Autodesk Inventor part; units mm, degrees
ref_plane "YZ Plane" through (0, 0, 0) normal (1, 0, 0) x (0, 1, 0)
ref_plane "XZ Plane" through (0, 0, 0) normal (0, 1, 0) x (-1, 0, 0)
ref_plane "XY Plane" through (0, 0, 0) normal (0, 0, 1) x (1, 0, 0)
sketch "Sketch2" plane through (0, 0, 0) normal (0, 1, 0) x (-1, 0, 0)
  line L0 (-30.2, -84) -> (30.2, -84)
  line L1 (30.2, -84) -> (30.2, 84)
  line L2 (30.2, 84) -> (-30.2, 84)
  line L3 (-30.2, 84) -> (-30.2, -84)
  line L4 (-30.2, -84) -> (30.2, 84) construction
  line L5 (30.2, -84) -> (-30.2, 84) construction
  point P0 (0, 0)
  dimension "d0" = 60.4
  dimension "d1" = 168
extrude "Extrusion1" add sketch "Sketch2" along normal blind 3
sketch "Sketch3" plane through (0, 3, 0) normal (0, 1, 0) x (1, 0, 0)
  line L0 (27.2, 81) -> (-27.2, 81)
  line L1 (-27.2, 81) -> (-27.2, -81)
  line L2 (-27.2, -81) -> (27.2, -81)
  line L3 (27.2, -81) -> (27.2, 81)
  line L4 (27.2, 81) -> (-27.2, -81) construction
  line L5 (-27.2, 81) -> (27.2, -81) construction
  line L6 (-30.2, 84) -> (-30.2, -84)
  line L7 (-30.2, -84) -> (30.2, -84)
  line L8 (24.2, 78) -> (-24.2, 78)
  line L9 (-24.2, 78) -> (-24.2, -78)
  line L10 (-24.2, -78) -> (24.2, -78)
  line L11 (24.2, -78) -> (24.2, 78)
  line L12 (24.2, 78) -> (-24.2, -78) construction
  line L13 (-24.2, 78) -> (24.2, -78) construction
  point P0 (0, 0)
  dimension "d4" = 3
  dimension "d5" = 3
  dimension "d6" = 3
  dimension "d7" = 3
extrude "Extrusion2" add sketch "Sketch3" along normal blind 30
fillet "Fillet1" radius 2 8 edges at (27.2, 18, 81) (-27.2, 18, 81) (-30.2, 1.5, 84) (30.2, 1.5, 84) (27.2, 18, -81) (-27.2, 18, -81) (30.2, 1.5, -84) (-30.2, 1.5, -84)
sketch "Sketch10" plane through (0, 3, 0) normal (0, 1, 0) x (1, 0, 0)
  line L0 (24.2, 78) -> (-24.2, 78)
  line L1 (-24.2, 78) -> (-24.2, -78)
  line L2 (-24.2, -78) -> (24.2, -78)
  line L3 (24.2, -78) -> (24.2, 78)
  line L4 (-24.2, -78) -> (24.2, -78)
  line L5 (24.2, -78) -> (24.2, -73.8)
  line L6 (24.2, -73.8) -> (-24.2, -73.8)
  line L7 (-24.2, -73.8) -> (-24.2, -78)
  line L8 (-24.2, -73.8) -> (24.2, -73.8)
  line L9 (24.2, -73.8) -> (24.2, 22.4)
  line L10 (24.2, 22.4) -> (-24.2, 22.4)
  line L11 (-24.2, 22.4) -> (-24.2, -73.8)
  line L12 (-24.2, 22.4) -> (24.2, 22.4)
  line L13 (24.2, 22.4) -> (24.2, 26.4)
  line L14 (24.2, 26.4) -> (-24.2, 26.4)
  line L15 (-24.2, 26.4) -> (-24.2, 22.4)
  point P0 (0, 0)
  point P1 (-24.2, 26.4)
  point P2 (-24.2, 22.4)
  dimension "d90" = 4.2
  dimension "d91" = 96.2
  dimension "d92" = 4
extrude "Extrusion9" add sketch "Sketch10" along normal blind 3 contours L3 L10 L1 L14 | L3 L2 L1 L6
sketch "Sketch11" plane through (0, 6, 0) normal (0, 1, 0) x (1, 0, 0)
  line L0 (-24.2, 22.4) -> (-24.2, 26.4)
  line L1 (-24.2, 22.4) -> (24.2, 22.4)
  line L2 (24.2, 26.4) -> (24.2, 22.4)
  line L3 (24.2, 26.4) -> (-24.2, 26.4)
  line L4 (-24.2, -78) -> (-24.2, -73.8)
  line L5 (24.2, -78) -> (-24.2, -78)
  line L6 (24.2, -73.8) -> (24.2, -78)
  line L7 (24.2, -73.8) -> (-24.2, -73.8)
  line L8 (24.2, 26.4) -> (-24.2, 26.4)
  line L9 (-24.2, 26.4) -> (24.2, 26.4)
  line L10 (24.2, 26.4) -> (24.2, 24.4)
  line L11 (24.2, 24.4) -> (-24.2, 24.4)
  line L12 (-24.2, 24.4) -> (-24.2, 26.4)
  line L13 (24.2, -73.8) -> (24.2, -78)
  line L14 (-24.2, -78) -> (24.2, -78)
  line L15 (24.2, -78) -> (24.2, -76)
  line L16 (24.2, -76) -> (-24.2, -76)
  line L17 (-24.2, -76) -> (-24.2, -78)
  point P0 (0, 0)
  point P1 (24.2, -72.6)
  point P2 (-24.2, -76)
  dimension "d95" = 2
  dimension "d120" = 2
extrude "Extrusion10" add sketch "Sketch11" along normal blind 1.6 contours L0 L3 L2 L11 | L4 L16 L6 L5
sketch "Sketch12" plane through (-25.2, 3, 81) normal (0, 0, 1) x (1, 0, 0)
  line L0 (-2, 30) -> (-2, 0)
  line L1 (0, 30) -> (50.4, 30)
  line L2 (-2, 30) -> (0, 30)
  line L3 (50.4, 30) -> (52.4, 30)
  line L4 (52.4, 0) -> (52.4, 30)
  line L5 (50.4, 0) -> (0, 0)
  line L6 (0, 0) -> (-2, 0)
  line L7 (52.4, 0) -> (50.4, 0)
  line L8 (15, 23.6) -> (23.06, 23.6)
  line L9 (23.06, 23.6) -> (23.06, 15)
  line L10 (23.06, 15) -> (15, 15)
  line L11 (15, 15) -> (15, 23.6)
  line L12 (27.34, 23.6) -> (35.4, 23.6)
  line L13 (35.4, 23.6) -> (35.4, 15)
  line L14 (35.4, 15) -> (27.34, 15)
  line L15 (27.34, 15) -> (27.34, 23.6)
  point P0 (25.2, -3)
  dimension "d116" = 8.06
  dimension "d117" = 8.6
  dimension "d118" = 15
  dimension "d119" = 17
  dimension "d121" = 8.06
  dimension "d122" = 8.6
  dimension "d123" = 15
  dimension "d124" = 17
extrude "Extrusion11" cut sketch "Sketch12" against normal blind 3 contours L8 L9 L10 L11 | L12 L13 L14 L15
sketch "Sketch13" plane through (0, 3, 0) normal (0, 1, 0) x (1, 0, 0)
  arc A0 (-28.2, 84) -> (-30.2, 82) centre (-28.2, 82) ccw
  line L0 (-30.2, 82) -> (-30.2, -82)
  arc A1 (-30.2, -82) -> (-28.2, -84) centre (-28.2, -82) ccw
  line L1 (-28.2, -84) -> (28.2, -84)
  arc A2 (28.2, -84) -> (30.2, -82) centre (28.2, -82) ccw
  line L2 (30.2, -82) -> (30.2, 82)
  arc A3 (30.2, 82) -> (28.2, 84) centre (28.2, 82) ccw
  line L3 (28.2, 84) -> (-28.2, 84)
  line L4 (-25.2, 81) -> (25.2, 81)
  arc A4 (27.2, 79) -> (25.2, 81) centre (25.2, 79) ccw
  line L5 (27.2, 79) -> (27.2, -79)
  arc A5 (25.2, -81) -> (27.2, -79) centre (25.2, -79) ccw
  line L6 (25.2, -81) -> (-25.2, -81)
  arc A6 (-27.2, -79) -> (-25.2, -81) centre (-25.2, -79) ccw
  line L7 (-27.2, -79) -> (-27.2, 79)
  arc A7 (-25.2, 81) -> (-27.2, 79) centre (-25.2, 79) ccw
  point P0 (0, 0)
extrude "Extrusion12" cut sketch "Sketch13" against normal blind 3
sketch "Sketch14" plane through (25.2, 33, -81) normal (0, 0, -1) x (-1, 0, 0)
  line L0 (1, -10) -> (49.4, -10)
  line L1 (49.4, -10) -> (49.4, -19.6)
  line L2 (49.4, -19.6) -> (1, -19.6)
  line L3 (1, -19.6) -> (1, -10)
  line L4 (52.4, -33) -> (52.4, 0)
  line L5 (-2, 0) -> (-2, -33)
  line L6 (50.4, 0) -> (50.4, -33)
  line L7 (50.4, -33) -> (0, -33)
  point P0 (25.2, -33)
  point P1 (50.4, -16.5)
  point P2 (49.4, -14.8)
  dimension "d127" = 9.6
  dimension "d128" = 3
  dimension "d129" = 3
  dimension "d140" = 23
extrude "Extrusion13" add sketch "Sketch14" along normal blind 6
sketch "Sketch15" plane through (-24.2, 13.4, -81) normal (-1, 0, 0) x (0, 0, 1)
  line L0 (0, 9.6) -> (-6, 9.6)
  line L1 (0, 9.6) -> (-3.4, 9.6)
  line L2 (-3.4, 9.6) -> (-3.4, 6.6)
  line L3 (-3.4, 6.6) -> (0, 6.6)
  line L4 (0, 6.6) -> (0, 9.6)
  line L5 (0, 9.6) -> (0, 0)
  line L6 (0, 9.6) -> (-6, 9.6)
  line L7 (-6, 0) -> (-6, 9.6)
  line L8 (0, 0) -> (-6, 0)
  line L9 (0, 0) -> (-3.4, 0)
  line L10 (-3.4, 0) -> (-3.4, 3)
  line L11 (-3.4, 3) -> (0, 3)
  line L12 (0, 3) -> (0, 0)
  point P0 (81, -13.4)
  point P1 (-3.4, 0)
  dimension "d133" = 3.4
  dimension "d134" = 3
  dimension "d135" = 3.4
  dimension "d136" = 3
extrude "Extrusion14" cut sketch "Sketch15" against normal up to surface (48.4 mm away) contours L4 L3 L2 L0 | L5 L8 L10 L11
fillet "Fillet8" radius 1 18 edges at (0, 23, -87) (0, 23, -84.4) (0, 13.4, -87) (0, 13.4, -84.4) (-24.2, 14.9, -84.4) (-24.2, 18.2, -87) (-24.2, 21.5, -84.4) (-24.2, 23, -85.7) (-24.2, 13.4, -85.7) (-24.2, 16.4, -82.7) (-24.2, 20, -82.7) (24.2, 20, -82.7) (24.2, 16.4, -82.7) (24.2, 14.9, -84.4) (24.2, 21.5, -84.4) (24.2, 23, -85.7) (24.2, 18.2, -87) (24.2, 13.4, -85.7)
sketch "Sketch16" plane through (-27.2, 0, -79) normal (-1, 0, 0) x (0, 0, 1)
  line L0 (147, 22.8) -> (134.9, 22.8)
  line L1 (134.9, 22.8) -> (134.9, 18)
  line L2 (134.9, 18) -> (147, 18)
  line L3 (147, 18) -> (147, 22.8)
  line L4 (160, 3) -> (160, 33)
  line L5 (152, 0) -> (0, 0)
  point P0 (79, 0)
  point P1 (154, 0)
  dimension "d141" = 12.1
  dimension "d142" = 4.8
  dimension "d143" = 13
  dimension "d144" = 18
extrude "Extrusion15" cut sketch "Sketch16" against normal through all
sketch "Sketch17" plane through (0, 33, 0) normal (0, 1, 0) x (1, 0, 0)
  arc A0 (-25.2, 81) -> (-27.2, 79) centre (-25.2, 79) ccw
  line L0 (-27.2, 79) -> (-27.2, -79)
  arc A1 (-27.2, -79) -> (-25.2, -81) centre (-25.2, -79) ccw
  line L1 (-25.2, -81) -> (25.2, -81)
  arc A2 (25.2, -81) -> (27.2, -79) centre (25.2, -79) ccw
  line L2 (27.2, -79) -> (27.2, 79)
  arc A3 (27.2, 79) -> (25.2, 81) centre (25.2, 79) ccw
  line L3 (25.2, 81) -> (-25.2, 81)
  line L4 (24.2, 78) -> (24.2, -78)
  line L5 (24.2, -78) -> (-24.2, -78)
  line L6 (-24.2, -78) -> (-24.2, 78)
  line L7 (-24.2, 78) -> (24.2, 78)
  line L8 (-26.2, 20) -> (-24.2, 20)
  line L9 (-24.2, 20) -> (-24.2, 16.6)
  line L10 (-24.2, 16.6) -> (-26.2, 16.6)
  line L11 (-26.2, 16.6) -> (-26.2, 20)
  line L12 (-24.2, -0.56) -> (-26.2, -0.56)
  line L13 (-26.2, -0.56) -> (-26.2, -3.96)
  line L14 (-26.2, -3.96) -> (-24.2, -3.96)
  line L15 (-24.2, -3.96) -> (-24.2, -0.56)
  line L16 (-24.2, 22.4) -> (-24.2, -73.8)
  line L17 (-24.2, -21.12) -> (-26.2, -21.12)
  line L18 (-26.2, -21.12) -> (-26.2, -24.52)
  line L19 (-26.2, -24.52) -> (-24.2, -24.52)
  line L20 (-24.2, -24.52) -> (-24.2, -21.12)
  line L21 (24.2, 20) -> (26.2, 20)
  line L22 (26.2, 20) -> (26.2, 16.6)
  line L23 (26.2, 16.6) -> (24.2, 16.6)
  line L24 (24.2, 16.6) -> (24.2, 20)
  line L25 (24.2, -0.56) -> (26.2, -0.56)
  line L26 (26.2, -0.56) -> (26.2, -3.96)
  line L27 (26.2, -3.96) -> (24.2, -3.96)
  line L28 (24.2, -3.96) -> (24.2, -0.56)
  line L29 (24.2, -21.12) -> (26.2, -21.12)
  line L30 (26.2, -21.12) -> (26.2, -24.52)
  line L31 (26.2, -24.52) -> (24.2, -24.52)
  line L32 (24.2, -24.52) -> (24.2, -21.12)
  point P0 (0, 0)
  point P1 (-24.2, 16.6)
  point P2 (24.2, 16.6)
  point P3 (24.2, -3.96)
  point P4 (24.2, -24.52)
  point P5 (-24.2, -24.52)
  point P6 (-24.2, -21.12)
  point P7 (-24.2, -3.96)
  dimension "d147" = 2
  dimension "d148" = 3.4
  dimension "d149" = 61
  dimension "d150" = 0
  dimension "d153" = 2
  dimension "d154" = 3.4
  dimension "d155" = 20.56
  dimension "d156" = 2
  dimension "d157" = 3.4
  dimension "d158" = 20.56
  dimension "d159" = 2
  dimension "d160" = 3.4
  dimension "d161" = 2
  dimension "d162" = 3.4
  dimension "d163" = 2
  dimension "d164" = 3.4
  dimension "d165" = 20.56
  dimension "d166" = 20.56
  dimension "d167" = 61
extrude "Extrusion16" cut sketch "Sketch17" against normal blind 3.2 contours L21 L22 L23 L4 | L25 L26 L27 L4 | L6 L10 L11 L8 | L29 L30 L31 L4 | L6 L14 L13 L12 | L6 L19 L18 L17
equation "\"d167\" = d149"
properties part number "module_switch" material "PC/ABS Plastic"
Input: part model. Units: mm. Frame: model coordinates. A direction names the side the tool comes from. Round coordinates to 2 decimals unless told otherwise and drop trailing zeros. Loops run counter-clockwise (first coordinate to the right, second up) from the corner with the lowest first, then second, coordinate; pieces in that order, holes last. Notation, with made-up numbers: (71, -17.5) -> (99, -17.5) arc R18 ccw to (99, 8.5) -> close; hole circle Ø9 at (53, 3.25). An arc over 180 degrees is marked (long way). Use one line per item in the form item = value. Start each with the question number.
Item 1: Section query C-C on z = 33.5. Return the cut outline in (x, y).
Item 2: Material intervals for L1, parallel to Z at x = 6, y = 4.5; L2, parallel to Z at x = -7, y = 7; L3, parallel to X at y = 28, z = 15, sorted ascending. Write a range as from..to.
Item 3: Contact query for flat-ended pins moving along their axis: pin 1 Ø1 at (x, z) = (1, 76.5) entering from +Y; pin 2 Ø1.6 at (x, z) = (25, -18.5) entering from +Y; pin 3 Ø1.5 at (x, z) = (15.5, 19.5) entering from +Y. Output: stop coordinate, or through.
Item 4: Set-up query: faces 1 (the face through (-26, 33, -24)), 2 (the face through (-24.2, 18, -84)), 3 (the face through (0, 4, 73.8)), 4 (the face through (-10.2, 22, 80)), 5 (the face through (26, 20, 55.9)). Return all of +Z, -Z, +X, -X, +Y, -Y with unobstructed straight access to the full face (end or side cutting, diameter ignored); none if empty.
Item 5: Mould query, pull axis Y, two halves, no side actions, for faces 6 (the face through (-2.14, 22, 80)), 7 (the face through (-26.2, 31, 23)), 8 (the face through (0, 0, 1)). Classes: pulls with the +Y half, pulls with the -Y half, needs draft (parallel to the pull), parting line crosses it, or undercut.
Ans:
q1.outline = (-27.2, 0) -> (27.2, 0) -> (27.2, 33) -> (24.2, 33) -> (24.2, 3) -> (-24.2, 3) -> (-24.2, 33) -> (-27.2, 33) -> close
q2.L1 = -81..-78, -26.4..-22.4, 73.8..81
q2.L2 = -81..-78, -26.4..-24.4, 76..81
q2.L3 = -27.2..-24.2, 24.2..27.2
q3.pin_1 = 7.6
q3.pin_2 = 29.8
q3.pin_3 = 3
q4.face_1 = +Z, -Z, +X, -X, +Y
q4.face_2 = -Z, -X, +Y, -Y
q4.face_3 = +Y
q4.face_4 = +Z
q4.face_5 = +X, -X
q5.face_6 = undercut
q5.face_7 = needs draft
q5.face_8 = pulls with the -Y half
